Input: dimensioned drawing with shaded views. Units: mm. Origin: part minimum x, y, z. A direction names the side the tool comes from. Coordinates: 2 decimals unless noted, no trailing zeros. Loops run counter-clockwise (first coordinate to the right, second up) from the corner with the lowest first, then second, coordinate; pieces in that order, holes last. Notation, with made-up numbers: (74.25, 18.25) - (118.25, 18.25) arc R36 cw to (118.25, 53.25) - close; hole circle Ø10 at (74.5, -18). An arc over 180 degrees is marked (long way). Write item = value, one per line. Start each with the question number.
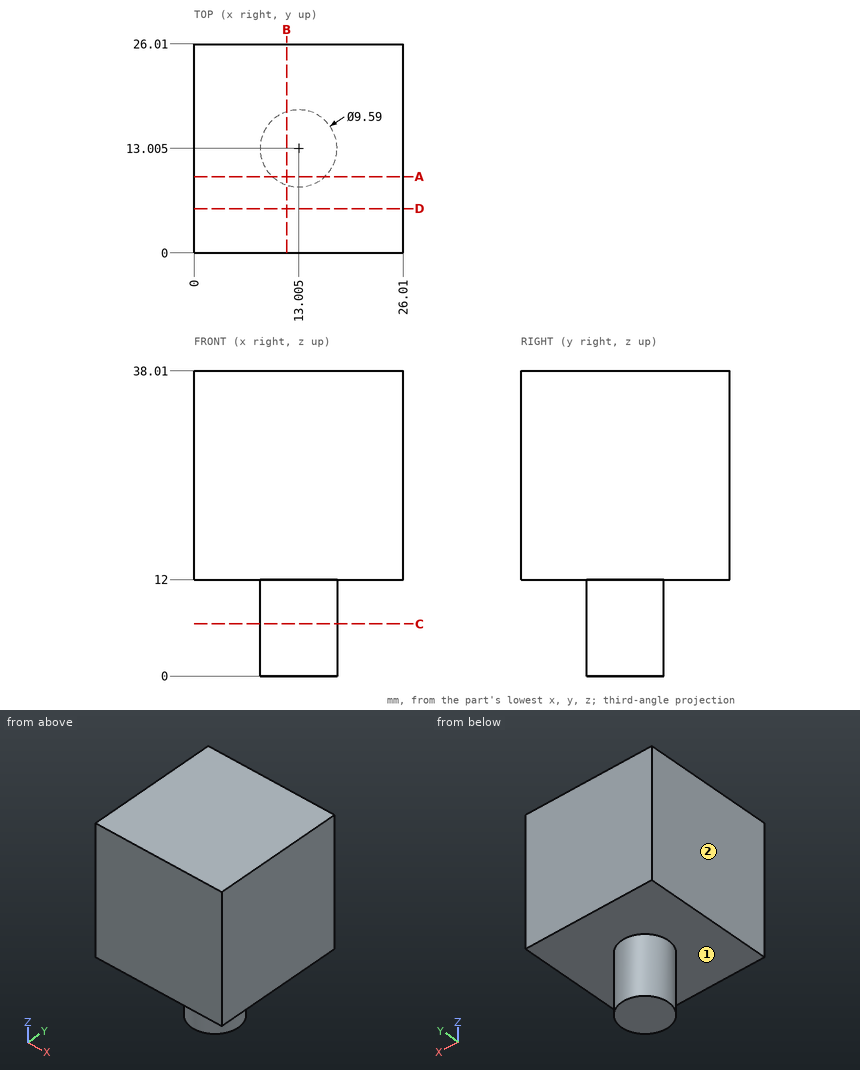
Item 1: Access query for the marked faces 1 and 2. Directions: +Z, -Z, +X, -X, +Y, -Y. A direction counts if a zero-diameter tool reaches every point of the face in a straight line with its end or side. Return the directions, or none.
Item 2: Ray query, line 1 (Z direction, x = 7, y = 24.5); line 2 (X direction, y = 11, z = 10). Return the intervals inside material, ascending.
Item 3: Pin query (flat end, axial travel): pin 1 (5 mm diameter, centred on x = 17.5, y = 7, fed in from -Z). Return the tip coordinate at first contact, or that it passes through.
Item 4: Cut plane D-D on y = 5.5. Return loops of the section in (x, z).
Item 5: Cut plane A-A on y = 9.5. Return loops of the section in (x, z).
Item 6: Cut plane B-B on x = 11.5. Return loops of the section in (y, z), plus the area to 3 significant figures.
Item 7: Cut plane C-C on z = 6.5. Return loops of the section in (x, y) (1 decimal).
Recorded:
q1.face_1 = -Z
q1.face_2 = +Z, -Z, -X, +Y, -Y
q2.line_1 = 12 to 38.01
q2.line_2 = 8.65 to 17.36
q3.pin_1 = 12
q4.outline = (0, 12) - (26.01, 12) - (26.01, 38.01) - (0, 38.01) - close
q5.outline = (0, 12) - (9.73, 12) - (9.73, 0) - (16.28, 0) - (16.28, 12) - (26.01, 12) - (26.01, 38.01) - (0, 38.01) - close
q6.outline = (0, 12) - (8.45, 12) - (8.45, 0) - (17.56, 0) - (17.56, 12) - (26.01, 12) - (26.01, 38.01) - (0, 38.01) - close
q6.area = 786 mm²
q7.outline = circle Ø9.6 at (13, 13)
